Geometry check sheet. Reference: drawing and pictorial views, mm from the part's lowest x, y, z. A direction names the side the tool comes from. Round coordinates to 2 decimals unless told otherwise and drop trailing zeros. Write each loop counter-clockwise with the first axis right and the second up, starting at its lowest first coordinate (ties: lowest second). Pieces come first, ordered by that corner, then holes. Notation, with made-up numbers: (21, -3.5) -> (31, -3.5) arc R14 cw to (31, 18.5) -> close; hole circle Ø3 at (29, 70.5). An arc over 180 degrees is marked (long way). Write item = value, one per line.
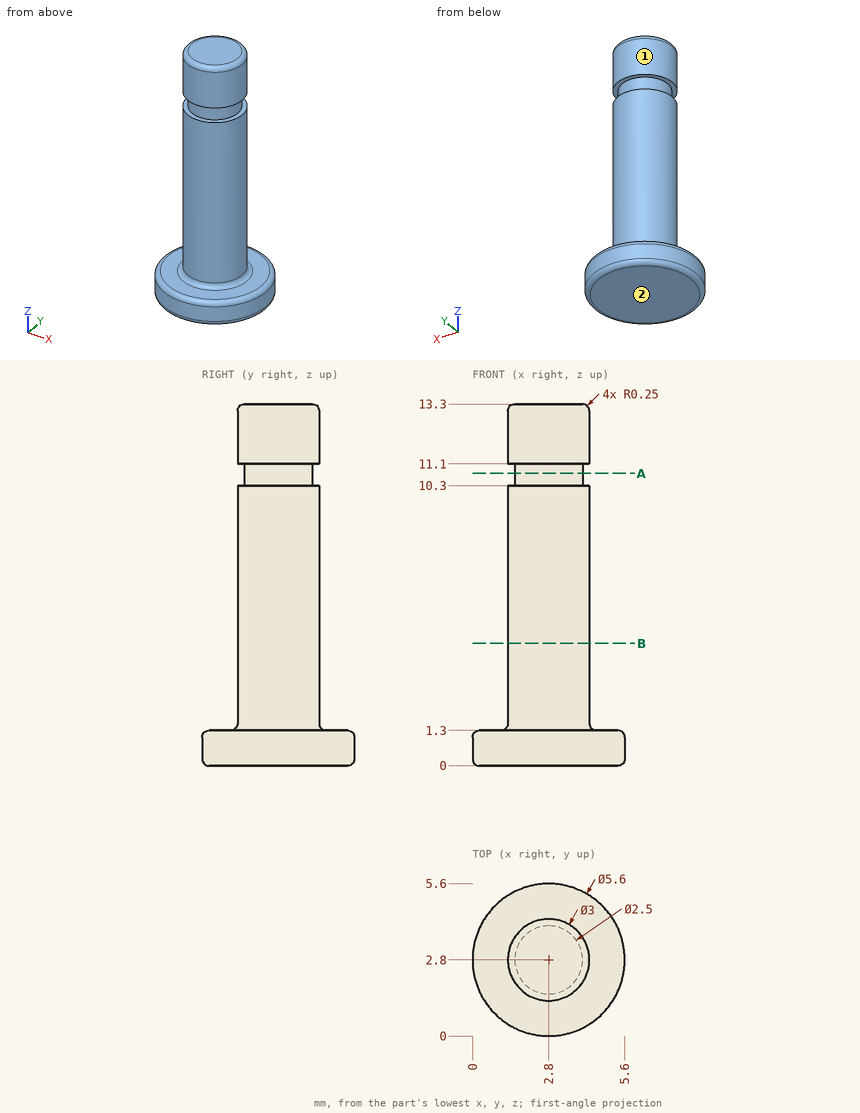
(1) Material ranges on L1, parallel to Z at x = 3, y = 0.6; L2, parallel to Y at x = 2.7, z = 4; L3, parallel to Z at x = 4.8, y = 0.95, recorded low to high. Write a range as [from, to].
Worked answers:
L1 = [0, 1.3]
L2 = [1.3, 4.3]
L3 = [0.07, 1.23]
(2) Access from +Z, -Z, +X, -X, +Y, -Y to the whole of each face (thin tool, end or side, straight path). Record for the marked faces 1 and 2.
Worked answers:
face_1 = +Z
face_2 = -Z, +X, -X, +Y, -Y
(3) Sectioned sample at B-B on z = 4.5. Enter the section's corners in (x, y).
Worked answers:
outline = circle Ø3 at (2.8, 2.8)
(4) Sectioned sample at A-A on z = 10.75. Enter the section's corners in (x, y), then the cut area to 3 significant figures.
Worked answers:
outline = circle Ø2.5 at (2.8, 2.8)
area = 4.91 mm²
(5) Go/stop test with flat-tipped pins: P1, Ø3, axis at y = 0.5, z = 8, coming from the -X side; P2, Ø1.5, axis at x = 0.5, y = 1.5, coming from the +Z side; P3, Ø2, axis at x = 1.5, z = 2, coming from the +Y side. Record where each tip stops, or that it passes through.
Worked answers:
P1 = 1.53
P2 = 1.3
P3 = 5.47
